from build123d import *

# Parameters (mm, degrees)
SKETCH1_R           = 6
SKETCH1_R_2         = 4
BOSS_EXTRUDE1_DEPTH = 1.75
SKETCH2_R           = 5.8
SKETCH2_R_2         = 4.2
CUT_EXTRUDE1_DEPTH  = 0.2


with BuildPart() as part:
    # Sketch1 → Boss-Extrude1 (new body, symmetric)
    with BuildSketch(Plane(origin=(0, 0, 0), x_dir=(1, 0, 0), z_dir=(0, 1, 0))):
        Circle(SKETCH1_R)
        Circle(SKETCH1_R_2, mode=Mode.SUBTRACT)
    extrude(amount=BOSS_EXTRUDE1_DEPTH, both=True)

    # Sketch2 → Cut-Extrude1 (cut)
    with BuildSketch(Plane(origin=(0, 1.75, 0), x_dir=(1, 0, 0), z_dir=(0, 1, 0))):
        Circle(SKETCH2_R)
        Circle(SKETCH2_R_2, mode=Mode.SUBTRACT)
    cut_extrude1 = extrude(amount=-CUT_EXTRUDE1_DEPTH, mode=Mode.SUBTRACT)

    # Mirror2: Cut-Extrude1 across plane
    add(cut_extrude1.mirror(Plane.ZX), mode=Mode.SUBTRACT)


solid = part.part
Source: CAD feature listing. Evaluate the final solid. Frame: model axes, mm. Coordinates: 2 decimals unless noted, no trailing zeros. Loops run counter-clockwise (first coordinate to the right, second up) from the corner with the lowest first, then second, coordinate; pieces in that order, holes last. Notation, with made-up numbers: (51, 84) - (60, 84) arc R18 cw to (60, 102) - close; hole circle Ø9 at (58.25, -2.75). An arc over 180 degrees is marked (long way). One line per item, written item: value. Start each with the question number.
1. Contact query for flat-ended pins moving along their axis: P1, Ø2, axis at y = -0.5, z = -2, coming from the -X side; P2, Ø1.5, axis at x = 2, y = 1, coming from the +Z side; P3, Ø2, axis at y = 0.5, z = -1.5, coming from the +X side. Output: stop coordinate, or through.
2. Ray query, L1, parallel to Z at x = 0, y = -1.6; L2, parallel to Z at x = 0, y = 0.4. Return the intervals inside material, ascending.
3. Mould query, pull axis Z, two halves, no side actions, for faces 1 (the flat face through (4, -1.55, -2)), 2 (the flat face through (4, 1.55, -2)), 3 (the cylindrical face through (-6, 0, 0)). Classes: pulls with the +Z half, pulls with the -Z half, needs draft (parallel to the pull), parting line crosses it, or undercut.
4. Section A-A (z = 0). Return the cut outline in (x, y), and give its area (3 significant figures).
5. Section C-C (y = -1.05). Return the cut outline in (x, z).
6. Section B-B (x = 0). Return the cut outline in (y, z).
Verdict:
1. P1: stops at x = -5.92
1. P2: stops at z = 5.87
1. P3: stops at x = 5.98
2. L1: z = -6 to -5.8, -4.2 to -4, 4 to 4.2, 5.8 to 6
2. L2: z = -6 to -4, 4 to 6
3. face 1: undercut
3. face 2: undercut
3. face 3: parting line crosses it
4. outline: (-6, -1.75) - (-5.8, -1.75) - (-5.8, -1.55) - (-4.2, -1.55) - (-4.2, -1.75) - (-4, -1.75) - (-4, 1.75) - (-4.2, 1.75) - (-4.2, 1.55) - (-5.8, 1.55) - (-5.8, 1.75) - (-6, 1.75) - close; (4, -1.75) - (4.2, -1.75) - (4.2, -1.55) - (5.8, -1.55) - (5.8, -1.75) - (6, -1.75) - (6, 1.75) - (5.8, 1.75) - (5.8, 1.55) - (4.2, 1.55) - (4.2, 1.75) - (4, 1.75) - close
4. area: 12.7 mm2
5. outline: circle Ø12 at (0, 0); hole circle Ø8 at (0, 0)
6. outline: (-1.75, -6) - (1.75, -6) - (1.75, -5.8) - (1.55, -5.8) - (1.55, -4.2) - (1.75, -4.2) - (1.75, -4) - (-1.75, -4) - (-1.75, -4.2) - (-1.55, -4.2) - (-1.55, -5.8) - (-1.75, -5.8) - close; (-1.75, 4) - (1.75, 4) - (1.75, 4.2) - (1.55, 4.2) - (1.55, 5.8) - (1.75, 5.8) - (1.75, 6) - (-1.75, 6) - (-1.75, 5.8) - (-1.55, 5.8) - (-1.55, 4.2) - (-1.75, 4.2) - close
